The drawing under review shows one solid part. Ordinate dimensions are in mm from its lowest x, y, z. A direction names the side the tool comes from. Coordinates: 2 decimals unless noted, no trailing zeros. Write each loop counter-clockwise with the first axis right and the second up, starting at its lowest first coordinate (ties: lowest second). Pieces come first, ordered by that corner, then holes.
1) Machinability: for the marked faces 4, 5 and 6, which of the approach directions +Z, -Z, +X, -X, +Y, -Y give a long, thin tool a straight path to every point of the face, cutting with its end or side? Answer none if there is none.
2) For line 1 (Y direction, x = 3.75, z = 19); line 2 (X direction, y = 11.5, z = 28); line 3 (X direction, y = 13, z = 13), list the stretches that pass through material, from the lowest coordinate up.
3) For P1, Ø4, axis at x = 19, z = 14.5, coming from the +Y side; P2, Ø2, axis at x = 27.5, z = 7.5, coming from the -Y side; P3, Ø3, axis at x = 35, y = 26.5, coming from the -Z side, all flat-tipped, find the tip position at first contact; note any pin that passes through.
4) Add section A-A, the plane z = 19. State the section outline as (x, y) points, then the cut area to 3 significant figures.
5) Add section B-B, the plane y = 16. State the section outline as (x, z) points.
6) Mouldability with a two-part tool opening along Y and no side actions: class the marked faces 1, 2 and 3 as released by +Y, released by -Y, zero draft, split by the parting line, or undercut.
7) Add section D-D, the plane y = 27.5. State the section outline as (x, z) points, then the cut area to 3 significant figures.
8) Add section C-C, the plane x = 26. State the section outline as (y, z) points, then the cut area to 3 significant figures.
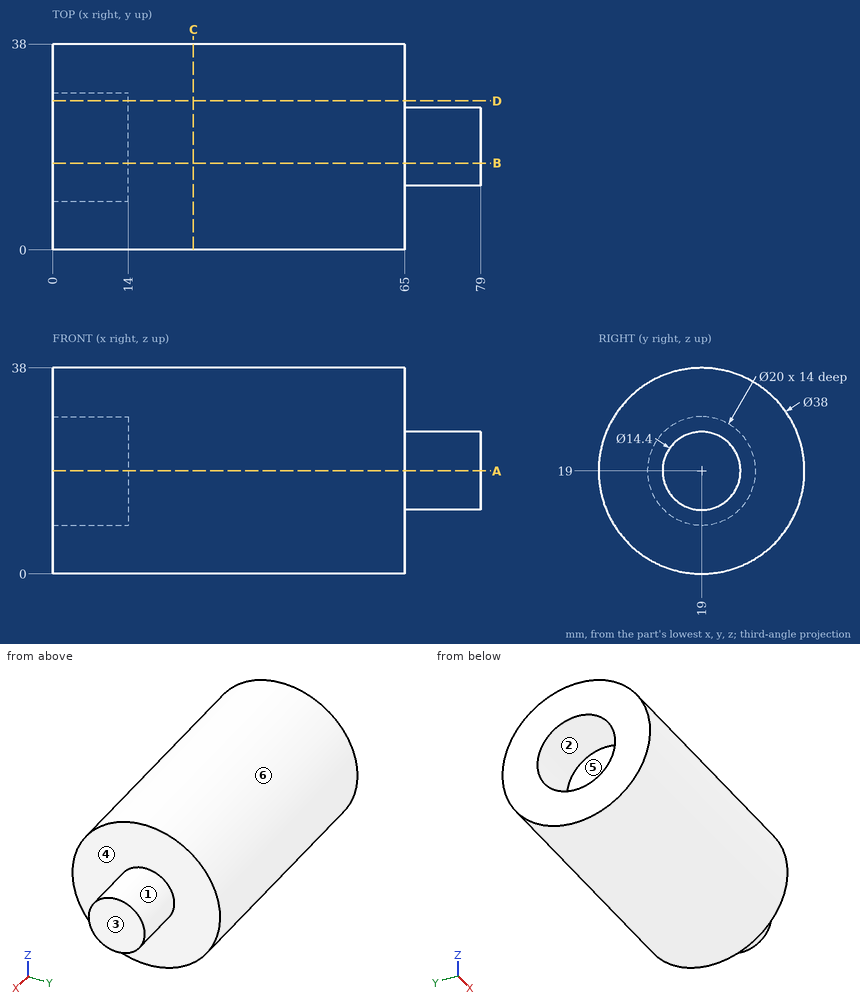
Geometry results:
1. face 4: +X
1. face 5: -X
1. face 6: +X, -X
2. line 1: y = 0 to 9, 29 to 38
2. line 2: x = 0 to 65
2. line 3: x = 14 to 65
3. P1: stops at y = 37.83
3. P2: stops at y = 3.16
3. P3: stops at z = 0.97
4. outline: (0, 0) - (65, 0) - (65, 11.8) - (79, 11.8) - (79, 26.2) - (65, 26.2) - (65, 38) - (0, 38) - (0, 29) - (14, 29) - (14, 9) - (0, 9) - close
4. area: 2,390 mm2
5. outline: (0, 0.24) - (65, 0.24) - (65, 12.45) - (79, 12.45) - (79, 25.55) - (65, 25.55) - (65, 37.76) - (0, 37.76) - (0, 28.54) - (14, 28.54) - (14, 9.46) - (0, 9.46) - close
6. face 1: split by the parting line
6. face 2: undercut
6. face 3: zero draft
7. outline: (0, 2.01) - (65, 2.01) - (65, 35.99) - (0, 35.99) - (0, 24.27) - (14, 24.27) - (14, 13.73) - (0, 13.73) - close
7. area: 2,060 mm2
8. outline: circle Ø38 at (19, 19)
8. area: 1,130 mm2
